Build history of the part. All positions in model axes, mm. A direction names the side the tool comes from. Round coordinates to 2 decimals unless told otherwise and drop trailing zeros. Loops run counter-clockwise (first coordinate to the right, second up) from the corner with the lowest first, then second, coordinate; pieces in that order, holes last.
from build123d import *

# Parameters (mm, degrees)
F1_DEPTH  = 6.25
F3_DEPTH  = 6.25
F5_DEPTH  = 6.25
F6_R      = 2.05
F6_R_2    = 3.05
F7_DEPTH  = 25
F8_R      = 2.05
F9_DEPTH  = 25
F10_R     = 2.05
F11_DEPTH = 25
F13_R     = 3.55
F14_DEPTH = 3
F15_R     = 3.55
F16_DEPTH = 3
F17_R     = 3.55
F17_R_2   = 4.55
F18_DEPTH = 3
F19_SIZE  = 5
F20_SIZE  = 3


with BuildPart() as f1:
    # F0 (on Top) → F1 (new body)
    with BuildSketch(Plane.XY):
        Polygon((4.1484118214, 32.5575917727), (-22.1015881786, 32.5575917727), (-22.1015881786, -13.6924082273), (24.1484118214, -13.6924082273), (24.1484118214, 12.5575917727), align=None)
    extrude(amount=F1_DEPTH)

    # F6 (on face) → F7 (cut)
    with BuildSketch(Plane.XY.offset(6.25)):
        with Locations((-5.8515881786, 22.5575917727)):
            Circle(F6_R)
        with Locations((-5.8515881786, 2.5575917727)):
            Circle(F6_R_2)
        with Locations((14.1484118214, 2.5575917727)):
            Circle(F6_R)
    extrude(amount=-F7_DEPTH, mode=Mode.SUBTRACT)


with BuildPart() as f3:
    # F2 (on face) → F3 (new body)
    with BuildSketch(Plane.XZ.offset(13.6924082273)):
        Polygon((-22.1015881786, 46.25), (-22.1015881786, 6.25), (24.1484118214, 6.25), (24.1484118214, 26.25), (-2.1015881786, 46.25), align=None)
    extrude(amount=-F3_DEPTH)

    # F8 (on face) → F9 (cut)
    with BuildSketch(Plane(origin=(0, -7.4424082273, 0), x_dir=(-1, 0, 0), z_dir=(0, 1, 0))):
        with Locations((5.8515881786, 16.25)):
            Circle(F8_R)
        with Locations((-14.1484118214, 16.25)):
            Circle(F8_R)
        with Locations((5.8515881786, 36.25)):
            Circle(F8_R)
    extrude(amount=-F9_DEPTH, mode=Mode.SUBTRACT)


with BuildPart() as f5:
    # F4 (on face) → F5 (new body)
    with BuildSketch(Plane(origin=(-22.1015881786, 0, 0), x_dir=(0, -1, 0), z_dir=(-1, 0, 0))):
        Polygon((-32.5575917727, 6.25), (7.4424082273, 6.25), (7.4424082273, 46.25), (-12.5575917727, 46.25), (-32.5575917727, 26.25), align=None)
    extrude(amount=-F5_DEPTH)

    # F10 (on face) → F11 (cut)
    with BuildSketch(Plane.YZ.offset(-15.8515881786)):
        with Locations((22.5575917727, 16.25)):
            Circle(F10_R)
        with Locations((2.5575917727, 16.25)):
            Circle(F10_R)
        with Locations((2.5575917727, 36.25)):
            Circle(F10_R)
    extrude(amount=-F11_DEPTH, mode=Mode.SUBTRACT)


with BuildPart() as f1_1:
    add(f1.part)

    # F12: union F3, F5
    add(f3.part)
    add(f5.part)

    # F13 (on face) → F14 (cut)
    with BuildSketch(Plane.XZ.offset(13.6924082273)):
        with Locations((-5.8515881786, 36.25)):
            Circle(F13_R)
        with Locations((14.1484118214, 16.25)):
            Circle(F13_R)
        with Locations((-5.8515881786, 16.25)):
            Circle(F13_R)
    extrude(amount=-F14_DEPTH, mode=Mode.SUBTRACT)

    # F15 (on face) → F16 (cut)
    with BuildSketch(Plane(origin=(-22.1015881786, 0, 0), x_dir=(0, -1, 0), z_dir=(-1, 0, 0))):
        with Locations((-2.5575917727, 36.25)):
            Circle(F15_R)
        with Locations((-2.5575917727, 16.25)):
            Circle(F15_R)
        with Locations((-22.5575917727, 16.25)):
            Circle(F15_R)
    extrude(amount=-F16_DEPTH, mode=Mode.SUBTRACT)

    # F17 (on face) → F18 (cut)
    with BuildSketch(Plane(origin=(0, 0, 0), x_dir=(1, 0, 0), z_dir=(0, 0, -1))):
        with Locations((-5.8515881786, -22.5575917727)):
            Circle(F17_R)
        with Locations((-5.8515881786, -2.5575917727)):
            Circle(F17_R_2)
        with Locations((14.1484118214, -2.5575917727)):
            Circle(F17_R)
    extrude(amount=-F18_DEPTH, mode=Mode.SUBTRACT)

    # F19
    f19_edges = [f1_1.edges().sort_by_distance(p)[0] for p in [
        (-22.101588, -13.692408, 23.125),
    ]]
    chamfer(f19_edges, length=F19_SIZE)

    # F20 (call 1 of 2: OpenCascade refuses the feature's edges together)
    f20_edges = [f1_1.edges().sort_by_distance(p)[0] for p in [
        (-9.601588, -13.692408, 46.25),
        (11.023412, -13.692408, 36.25),
        (24.148412, -13.692408, 13.125),
    ]]
    chamfer(f20_edges, length=F20_SIZE)

    # F20#2 (call 2 of 2)
    f20_2_edges = [f1_1.edges().sort_by_distance(p)[0] for p in [
        (-22.101588, 1.932592, 46.25),
        (-22.101588, 22.557592, 36.25),
        (-22.101588, 32.557592, 13.125),
    ]]
    chamfer(f20_2_edges, length=F20_SIZE)


solid = f1_1.part
(1) Pin check, flat tips, straight feed: P1, Ø6.5, axis at x = -5.85, y = 22.56, coming from the +Z side; P2, Ø6.5, axis at x = -5.85, z = 36.25, coming from the -Y side; P3, Ø5.5, axis at x = -5.5, y = 22, coming from the -Z side; P4, Ø4, axis at x = 11.5, z = 40.5, coming from the -Y side. Stop position of each tip, or through.
Responses:
P1: stops at z = 6.25
P2: stops at y = -10.69
P3: stops at z = 3
P4: passes through
(2) Slice it at A-A on z = 8.5. List the corners of the cut face in (x, y).
Responses:
outline: (-22.1, -8.69) - (-17.1, -13.69) - (21.15, -13.69) - (24.15, -10.69) - (24.15, -7.44) - (-15.85, -7.44) - (-15.85, 32.56) - (-19.1, 32.56) - (-22.1, 29.56) - close
(3) Probe line 1 (Y direction, x = -19, z = 16); line 2 (Y direction, x = -7.5, z = 5); line 3 (X direction, y = 14, z = 31). List the from-to ranges inside material, lowest first.
Responses:
line 1: y = -11.79 to 0.52, 4.59 to 20.52, 24.59 to 32.56
line 2: y = -13.69 to -0.01, 5.12 to 21.34, 23.78 to 32.56
line 3: x = -22.1 to -15.85
(4) Which spindle directions (+Z, -Z, +X, -X, +Y, -Y) get a long thin tool onto all of the face, cutting with end or side? Do faces 1 (the face through (-3.943, 19.564, 1.479)), 2 (the face through (-17.454, 2.291, 38.283)), 3 (the face through (-3.94, -12.21, 19.24)), 4 (the face through (-20.623, 20.649, 19.243)), 5 (the face through (11.21, -9.09, 36.11)). Say none if no direction does.
Responses:
face 1: -Z
face 2: +X, -X
face 3: -Y
face 4: -X
face 5: +Z, +X, +Y, -Y
(5) Slice it at C-C on x = 5. List the corners of the cut face in (y, z).
Responses:
outline: (-13.69, 0) - (31.71, 0) - (31.71, 6.25) - (-7.44, 6.25) - (-7.44, 40.84) - (-10.69, 40.84) - (-13.69, 37.07) - close
(6) Slice it at B-B on z = 36.25. List the corners of the cut face in (x, y).
Responses:
outline: (-22.1, -8.69) - (-17.1, -13.69) - (-9.4, -13.69) - (-9.4, -10.69) - (-7.9, -10.69) - (-7.9, -7.44) - (-15.85, -7.44) - (-15.85, 0.51) - (-19.1, 0.51) - (-19.1, -0.99) - (-22.1, -0.99) - close; (-22.1, 6.11) - (-19.1, 6.11) - (-19.1, 4.61) - (-15.85, 4.61) - (-15.85, 22.56) - (-19.1, 22.56) - (-22.1, 18.31) - close; (-3.8, -10.69) - (-2.3, -10.69) - (-2.3, -13.69) - (6.07, -13.69) - (11.02, -10.69) - (11.02, -7.44) - (-3.8, -7.44) - close
(7) Slice it at D-D on y = 3.5. Count the separate pieces of the cut face and the enclosed holes in it, plus the area to 3 significant figures.
Responses:
separate pieces: 5
enclosed holes: 0
area: 392 mm2
(8) Pull direction Z, two halves, no side cores. Call faces 6 (the face through (-17, -3, 46.25)), 7 (the face through (4, -7.442, 22)), 8 (the face through (-4, -10.692, 15)): +Z half, -Z half, draft (parallel to the pull), parting line (faces both ways), or undercut.
Responses:
face 6: +Z half
face 7: draft
face 8: undercut
